Here's how the part is built. I have some questions about the finished solid (model axes, mm). Give positions to 0.01 mm unless a question says otherwise; leave off trailing zeros. Loops run counter-clockwise (first coordinate to the right, second up) from the corner with the lowest first, then second, coordinate; pieces in that order, holes last. Notation, with made-up numbers: (-1.75, 44) - (36.25, 44) arc R25 cw to (36.25, 72) - close; hole circle Ø5 at (31.5, -10). An arc over 180 degrees is marked (long way). Use one line per item in the form item = value.
from build123d import *

# Parameters (mm, degrees)
SKETCH1_W            = 350
SKETCH1_H            = 347
BASE_FLANGE1_DEPTH   = 1.51892
M3_CLEARANCE_HOLE1_D = 3.6
M4_CLEARANCE_HOLE1_D = 4.8
SKETCH13_R           = 8.5
SKETCH13_R_2         = 1.375
CUT_EXTRUDE1_DEPTH   = 1.51892
SKETCH41_W           = 347
SKETCH41_H           = 1.51892
BOSS_EXTRUDE4_DEPTH  = 1.905
SKETCH42_W           = 347
SKETCH42_H           = 1.51892
BOSS_EXTRUDE5_DEPTH  = 1.905
CUT_EXTRUDE2_DEPTH   = 1.51892
BOSS_EXTRUDE6_DEPTH  = 1.51892
CLEARANCE_HOLE2_D    = 3.4
FILLET2_R            = 5
SKETCH50_OUTSIDE_W   = 455.91
SKETCH50_OUTSIDE_H   = 456.1
SKETCH50_OUTSIDE_W_2 = 240
SKETCH50_OUTSIDE_H_2 = 240
CUT_EXTRUDE3_DEPTH   = 1.51892
M5_CLEARANCE_HOLE1_D = 5.5


# Sheet-metal steps are written as plain solids
with BuildPart() as part:
    # Sketch1 → Base-Flange1 (new body)
    with BuildSketch(Plane(origin=(0, 0, 0), x_dir=(1, 0, 0), z_dir=(0, 1, 0))):
        with Locations((0, 13.5)):
            Rectangle(SKETCH1_W, SKETCH1_H)
    extrude(amount=-BASE_FLANGE1_DEPTH)

    # M3 Clearance Hole1 (through all)
    with Locations(Plane(origin=(0, 0, 0), x_dir=(1, 0, 0), z_dir=(0, 1, 0))):
        with Locations((-105, 105), (105, 105), (105, -105), (-105, -105)):
            Hole(M3_CLEARANCE_HOLE1_D / 2)

    # M4 Clearance Hole1 (through all)
    with Locations(Plane(origin=(0, -1.51892, 0), x_dir=(-1, 0, 0), z_dir=(0, -1, 0))):
        with Locations((167.5, 146.5), (167.5, 169), (-167.5, 146.5), (-167.5, 169), (-167.5, -149), (-167.5, -126.5), (167.5, -149), (167.5, -126.5)):
            Hole(M4_CLEARANCE_HOLE1_D / 2)

    # Sketch13 → Cut-Extrude1 (cut)
    with BuildSketch(Plane(origin=(0, 0, 0), x_dir=(1, 0, 0), z_dir=(0, 1, 0))):
        with Locations(Location((0, 170, 0), (0, 0, 270))):
            Circle(SKETCH13_R)
        with Locations(Location((-11.825, 170, 0), (0, 0, 270))):
            Circle(SKETCH13_R_2)
        with Locations(Location((11.825, 170, 0), (0, 0, 270))):
            Circle(SKETCH13_R_2)
    extrude(amount=-CUT_EXTRUDE1_DEPTH, mode=Mode.SUBTRACT)

    # Sketch41 → Boss-Extrude4 (add)
    with BuildSketch(Plane(origin=(175, 0, 0), x_dir=(0, 0, -1), z_dir=(1, 0, 0))):
        with Locations((13.5, -0.75946)):
            Rectangle(SKETCH41_W, SKETCH41_H)
    extrude(amount=BOSS_EXTRUDE4_DEPTH)

    # Sketch42 → Boss-Extrude5 (add)
    with BuildSketch(Plane.ZY.offset(175)):
        with Locations((-13.5, -0.75946)):
            Rectangle(SKETCH42_W, SKETCH42_H)
    extrude(amount=BOSS_EXTRUDE5_DEPTH)

    # Sketch43 → Cut-Extrude2 (cut)
    with BuildSketch(Plane(origin=(0, 0, 0), x_dir=(1, 0, 0), z_dir=(0, 1, 0))):
        Polygon((-176.905, -120), (-120, -63.095), (-120, 80.095), (-176.905, 137), align=None)
        Polygon((-156.905, 177), (-99.905, 120), (-42.952595893, 120), (-25, 187), (-176.905, 187), (-176.905, 177), align=None)
        Polygon((25, 187), (42.952595893, 120), (99.905, 120), (156.905, 177), (176.905, 177), (176.905, 187), align=None)
        Polygon((120, 80.095), (120, -63.095), (176.905, -120), (176.905, 137), align=None)
        Polygon((116.905, -120), (-116.905, -120), (-156.905, -160), (156.905, -160), align=None)
    extrude(amount=-CUT_EXTRUDE2_DEPTH, mode=Mode.SUBTRACT)

    # Sketch45 → Boss-Extrude6 (add)
    with BuildSketch(Plane(origin=(0, 0, 0), x_dir=(1, 0, 0), z_dir=(0, 1, 0))):
        Polygon((-25, 187), (-23.124355653, 194), (23.124355653, 194), (25, 187), align=None)
    extrude(amount=-BOSS_EXTRUDE6_DEPTH)

    # Clearance Hole2 (through all)
    with Locations(Plane(origin=(0, 0, 0), x_dir=(1, 0, 0), z_dir=(0, 1, 0))):
        with Locations((-9.525, 188), (9.525, 188)):
            Hole(CLEARANCE_HOLE2_D / 2)

    # Fillet2
    fillet2_edges = [part.edges().sort_by_distance(p)[0] for p in [
        (176.905, -0.75946, 160),
        (-176.905, -0.75946, 160),
        (176.905, -0.75946, -177),
        (42.952595893, -0.75946, -120),
        (99.905, -0.75946, -120),
        (156.905, -0.75946, -177),
        (176.905, -0.75946, 120),
        (176.905, -0.75946, -137),
        (120, -0.75946, -80.095),
        (120, -0.75946, 63.095),
        (-176.905, -0.75946, -137),
        (-176.905, -0.75946, 120),
        (-120, -0.75946, 63.095),
        (-120, -0.75946, -80.095),
        (-176.905, -0.75946, -177),
        (-156.905, -0.75946, -177),
        (-99.905, -0.75946, -120),
        (-42.952595893, -0.75946, -120),
        (-156.905, -0.75946, 160),
        (156.905, -0.75946, 160),
        (116.905, -0.75946, 120),
        (-116.905, -0.75946, 120),
        (-23.124355653, -0.75946, -194),
        (23.124355653, -0.75946, -194),
    ]]
    fillet(fillet2_edges, radius=FILLET2_R)

    # Sketch50 outside → Cut-Extrude3 (cut)
    with BuildSketch(Plane(origin=(0, 0, 0), x_dir=(1, 0, 0), z_dir=(0, 1, 0))):
        with Locations((0, 17)):
            Rectangle(SKETCH50_OUTSIDE_W, SKETCH50_OUTSIDE_H)
        Rectangle(SKETCH50_OUTSIDE_W_2, SKETCH50_OUTSIDE_H_2, mode=Mode.SUBTRACT)
    extrude(amount=-CUT_EXTRUDE3_DEPTH, mode=Mode.SUBTRACT)

    # M5 Clearance Hole1 (through all)
    with Locations(Plane(origin=(0, 0, 0), x_dir=(1, 0, 0), z_dir=(0, 1, 0))):
        with Locations((-114.3, 114.3), (114.3, 114.3), (114.3, -114.3), (-114.3, -114.3), (-114.3, 0), (0, 114.3), (114.3, 0), (0, -114.3)):
            Hole(M5_CLEARANCE_HOLE1_D / 2)


solid = part.part
(1) If we section it at D-D (z = 0): List the corners of the cut face in (x, y) for me.
Geometry says:
outline = (-120, -1.52) - (-117.05, -1.52) - (-117.05, 0) - (-120, 0) - close; (-111.55, -1.52) - (111.55, -1.52) - (111.55, 0) - (-111.55, 0) - close; (117.05, -1.52) - (120, -1.52) - (120, 0) - (117.05, 0) - close
(2) If we section it at A-A (x = -114.3): List the corners of the cut face in (y, z) for me.
Geometry says:
outline = (-1.52, -120) - (0, -120) - (0, -117.05) - (-1.52, -117.05) - close; (-1.52, -111.55) - (0, -111.55) - (0, -2.75) - (-1.52, -2.75) - close; (-1.52, 2.75) - (0, 2.75) - (0, 111.55) - (-1.52, 111.55) - close; (-1.52, 117.05) - (0, 117.05) - (0, 120) - (-1.52, 120) - close
(3) If we section it at B-B (z = 114.3): List the corners of the cut face in (x, y) for me.
Geometry says:
outline = (-120, -1.52) - (-117.05, -1.52) - (-117.05, 0) - (-120, 0) - close; (-111.55, -1.52) - (-2.75, -1.52) - (-2.75, 0) - (-111.55, 0) - close; (2.75, -1.52) - (111.55, -1.52) - (111.55, 0) - (2.75, 0) - close; (117.05, -1.52) - (120, -1.52) - (120, 0) - (117.05, 0) - close
(4) If I drill on probe 1 along Z at (x, y) = (0, -0.75); probe 2 along Z at (x, y) = (-114.3, -0.5); probe 3 along X at (y, z) = (-0.35, -103.5), over which ranges is the centre line in solid material (lowest first)?
Geometry says:
probe_1 = -120 to -117.05, -111.55 to 111.55, 117.05 to 120
probe_2 = -120 to -117.05, -111.55 to -2.75, 2.75 to 111.55, 117.05 to 120
probe_3 = -120 to -105.99, -104.01 to 104.01, 105.99 to 120
(5) Thinking about a two-plate mould opening in Z: for faces 1 (the flat face through (2, 0, -2)), 2 (the cylindrical face through (0.596, -0.77, -111.615)), which applies, pulls with the +Z half, pulls with the -Z half, needs draft (parallel to the pull), parting line crosses it, or undercut?
Geometry says:
face_1 = needs draft
face_2 = undercut
(6) If we section it at C-C (x = 0): List the corners of the cut face in (y, z) for me.
Geometry says:
outline = (-1.52, -120) - (0, -120) - (0, -117.05) - (-1.52, -117.05) - close; (-1.52, -111.55) - (0, -111.55) - (0, 111.55) - (-1.52, 111.55) - close; (-1.52, 117.05) - (0, 117.05) - (0, 120) - (-1.52, 120) - close
(7) For P1, Ø4, axis at x = -105, z = 105, coming from the -Y side, with a flat end and sliding along its axis, tell me the tip position at first contact or that it passes through.
Geometry says:
P1 = -1.52
